```python
from build123d import *

# Parameters (mm, degrees)
BOSS_EXTRUDE1_DEPTH = 4.5


with BuildPart() as part:
    # Sketch1 → Boss-Extrude1 (new body, symmetric)
    with BuildSketch(Plane.XY):
        with BuildLine():
            Line((0.913333333, 13.669521653), (-94.66, 20.055283593))
            ThreePointArc((-94.66, 20.055283593), (-115.881273585, -2.957187963), (-88.88100799, -18.797072984))
            Line((-88.88100799, -18.797072984), (-50.656340302, -4.32029226))
            ThreePointArc((-50.656340302, -4.32029226), (-48.560454158, -3.855095369), (-46.418644181, -4.002733114))
            Line((-46.418644181, -4.002733114), (-2.888609962, -13.392010024))
            ThreePointArc((-2.888609962, -13.392010024), (13.566762828, -1.906028956), (0.913333333, 13.669521653))
        make_face()
        with BuildLine():
            Line((-51.010519009, -3.385114499), (-89.235186697, -17.861895224))
            ThreePointArc((-89.235186697, -17.861895224), (-114.892155496, -2.810064183), (-94.726666667, 19.05750829))
            Line((-94.726666667, 19.05750829), (0.846666667, 12.67174635))
            ThreePointArc((0.846666667, 12.67174635), (12.576488169, -1.766902755), (-2.67776252, -12.414491044))
            Line((-2.67776252, -12.414491044), (-46.207796739, -3.025214134))
            ThreePointArc((-46.207796739, -3.025214134), (-48.635181379, -2.857891357), (-51.010519009, -3.385114499))
        make_face(mode=Mode.SUBTRACT)
    extrude(amount=BOSS_EXTRUDE1_DEPTH, both=True)


solid = part.part
```
CAD build for the part. Positions are in the model's coordinates, mm. A direction names the side the tool comes from. Coordinates: 2 decimals unless noted, no trailing zeros. Write each loop counter-clockwise with the first axis right and the second up, starting at its lowest first coordinate (ties: lowest second). Pieces come first, ordered by that corner, then holes. Notation, with made-up numbers: (-15, 49) -> (-7, 49) arc R14 cw to (-7, 59) -> close; hole circle Ø4 at (88.25, 76). An arc over 180 degrees is marked (long way). Use CSV: the item, a comma, the result in double quotes. Start each with the question number.
Item 1: Two-plate mould, pull along Y, no slides. Class faces 1 (the cylindrical face through (-114.816, -3.281, 0.063)), 2 (the cylindrical face through (-48.591, -3.857, 0.063)), 3 (the cylindrical face through (-116, -2, 0)): +Y half, -Y half, draft (parallel to the pull), parting line (faces both ways), or undercut.
Item 2: Band-saw the part on A-A, the plane y = 0. Write the cut outline in (x, z).
Item 3: Tool access for faces 4 (the flat face through (-70.04, -11.66, 0.06)), 5 (the flat face through (-24.138, -7.786, 0.063)), 6 (the flat face through (-52, -4, 4.5)): list every direction of +Z, -Z, +X, -X, +Y, -Y with a clear straight run to the whole face (end or side of a thin tool).
Item 4: Drop flat-ended pins along their axis: P1, Ø2, axis at x = -47, z = -2, coming from the -Y side; P2, Ø3, axis at x = -64, y = -5, coming from the +Z side (1 decimal); P3, Ø4, axis at y = -6, z = 0.5, coming from the +X side; P4, Ø5, axis at y = 7, z = 3.5, coming from the -X side. Give the stop position or say it passes through.
Item 5: Band-saw the part on D-D, the plane y = -7.5. Write the cut outline in (x, z), plus the area to 3 significant figures.
Item 6: Wall check: probe 1 along Y at (x, z) = (-96, -1); probe 2 along X at (y, z) = (0, -2.5); probe 3 along Y at (x, z) = (-63.5, 3.5). Give the ranges that are in metal, low to high.
Item 7: Band-saw the part on B-B, the plane x = -96. Write the cut outline in (y, z).
Item 8: Band-saw the part on C-C, the plane z = -0.5. Write the cut outline in (x, y).
Response values:
1,face 1,"undercut"
1,face 2,"-Y half"
1,face 3,"parting line"
2,outline,"(-116.1, -4.5) -> (-115.1, -4.5) -> (-115.1, 4.5) -> (-116.1, 4.5) -> close; (12.7, -4.5) -> (13.7, -4.5) -> (13.7, 4.5) -> (12.7, 4.5) -> close"
3,face 4,"+Z, -Z, -Y"
3,face 5,"+Z, -Z"
3,face 6,"+Z, +X, -X, +Y, -Y"
4,P1,"stops at y = -4.09"
4,P2,"passes through"
4,P3,"stops at x = 13.1"
4,P4,"stops at x = -115.59"
5,outline,"(-114.65, -4.5) -> (-113.57, -4.5) -> (-113.57, 4.5) -> (-114.65, 4.5) -> close; (-61.88, -4.5) -> (-59.05, -4.5) -> (-59.05, 4.5) -> (-61.88, 4.5) -> close; (-30.2, -4.5) -> (-25.46, -4.5) -> (-25.46, 4.5) -> (-30.2, 4.5) -> close; (10.25, -4.5) -> (11.46, -4.5) -> (11.46, 4.5) -> (10.25, 4.5) -> close"
5,area,"88.8 mm2"
6,probe 1,"y = -20.1 to -19.1, 19.1 to 20.1"
6,probe 2,"x = -116.1 to -115.1, 12.7 to 13.7"
6,probe 3,"y = -9.18 to -8.12, 16.97 to 17.97"
7,outline,"(-20.1, -4.5) -> (-19.1, -4.5) -> (-19.1, 4.5) -> (-20.1, 4.5) -> close; (19.1, -4.5) -> (20.1, -4.5) -> (20.1, 4.5) -> (19.1, 4.5) -> close"
8,outline,"(-94.66, 20.06) arc R20.1 ccw (long way) to (-88.88, -18.8) -> (-50.66, -4.32) arc R7.5 cw to (-46.42, -4) -> (-2.89, -13.39) arc R13.7 ccw (long way) to (0.91, 13.67) -> close; hole (-94.73, 19.06) arc R19.1 ccw (long way) to (-89.24, -17.86) -> (-51.01, -3.39) arc R8.5 cw to (-46.21, -3.03) -> (-2.68, -12.41) arc R12.7 ccw (long way) to (0.85, 12.67) -> close"
